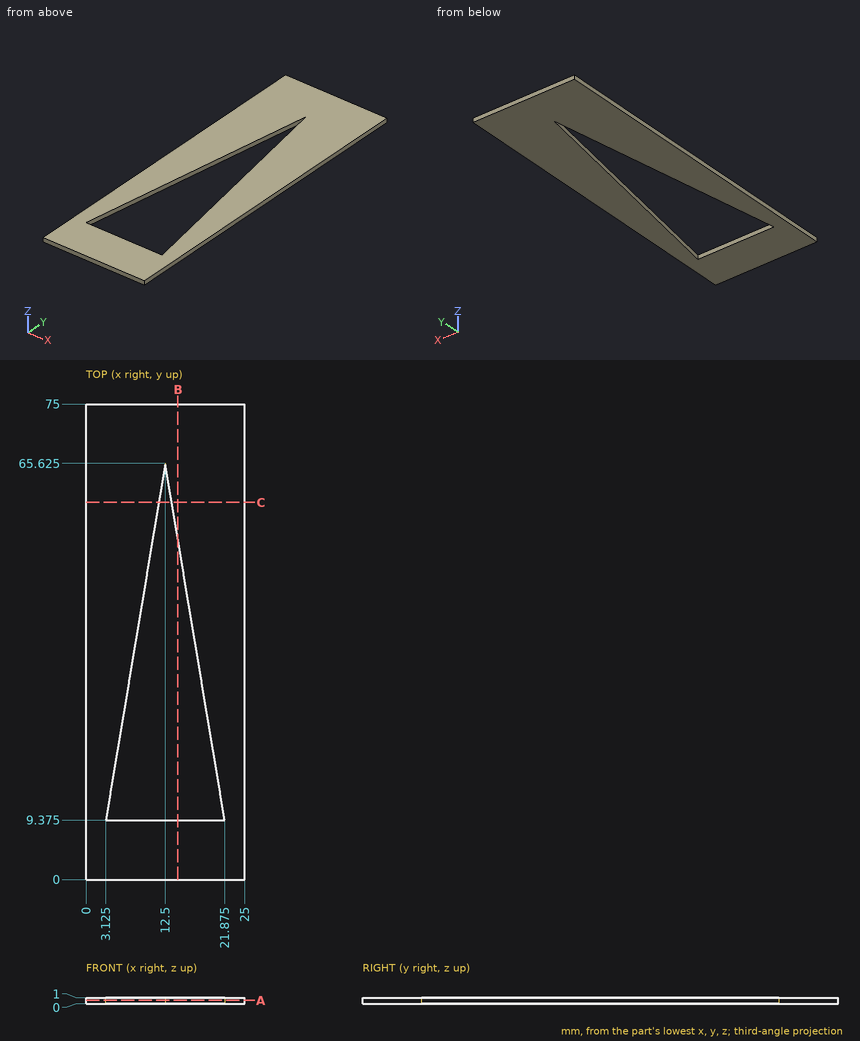
Could you check a few things on this drawing? It's one solid part, dimensions in mm from its lowest x, y, z. Round coordinates to 2 decimals unless told otherwise and drop trailing zeros. Loops run counter-clockwise (first coordinate to the right, second up) from the corner with the lowest first, then second, coordinate; pieces in that order, holes last. Notation, with made-up numbers: M 47.5,-6.5 L 104.5,-6.5 A26 cw 104.5,28.5 Z; hole C 20.5,16 d2. An arc over 180 degrees is marked long. Write each question's results on one line, items separated by ' | '. Start each with the question number.
(1) Will this pin go through, and if not, where does the flat tip stop? P1, Ø10, axis at x = 12.5, y = 28, coming from the +Z side.
(2) If I drill on probe 1 along X at (y, z) = (40, 0.1); probe 2 along X at (y, z) = (12, 0.75), over which ranges is the centre line in solid material (lowest first)? Write a range as from..to.
(3) I want a section at B-B (x = 14.5). Please give me the cut outline in (y, z) (3 decimals), then the cut area to 4 significant figures.
(4) I want a section at C-C (y = 59.5). Please give me the cut outline in (x, z).
(5) I want a section at A-A (z = 0.55). Please give me the cut outline in (x, y) (3 decimals), then the cut area to 3 significant figures.
Solved:
1) P1: passes through
2) probe 1: x = 0..8.23, 16.77..25 | probe 2: x = 0..3.56, 21.44..25
3) outline: M 0,0 L 9.375,0 L 9.375,1 L 0,1 Z; M 53.625,0 L 75,0 L 75,1 L 53.625,1 Z | area: 30.75 mm²
4) outline: M 0,0 L 11.48,0 L 11.48,1 L 0,1 Z; M 13.52,0 L 25,0 L 25,1 L 13.52,1 Z
5) outline: M 0,0 L 25,0 L 25,75 L 0,75 Z; hole M 3.125,9.375 L 21.875,9.375 L 12.5,65.625 Z | area: 1,350 mm²
